The listing builds one solid part. Answer for the finished solid, in the listing's coordinates (mm). Face numbers are marked on the shaded views. A direction names the side the tool comes from. Coordinates: 2 decimals unless noted, no trailing zeros. Write each loop counter-clockwise with the first axis right and the second up, starting at its lowest first coordinate (ties: lowest second). Pieces come first, ordered by that corner, then holes.
(1) Given P1, Ø1, axis at y = -0.5, z = 6.5, coming from the +X side; P2, Ø6, axis at y = -5.5, z = 15, coming from the -X side; P3, Ø4, axis at x = 13, z = 8.5, coming from the +Y side, each flat-ended and moving along its own axis, determine where each tip first touches the part or whether it passes through.
(2) Which of the six approach directions +Z, -Z, +X, -X, +Y, -Y give full straight-line access (tool end or side, diameter ignored) to the marked faces 1 and 2?
(3) Straight lines are drawn through the part: line 1 (Y direction, x = 23.25, z = 12.5); line 2 (Y direction, x = 13, z = 4.75); line 3 (X direction, y = 11.5, z = 13.75). For each, find the intervals that lie inside material, in ascending order.
(4) The part is cut by section B-B on x = 23.75. Determine the outline of the cut face in (y, z).
(5) The part is cut by section A-A on z = 2.75. Determine the outline of the cut face in (x, y).
(6) The part is cut by section C-C on y = 12.5. Determine the outline of the cut face in (x, z), plus the area to 3 significant figures.
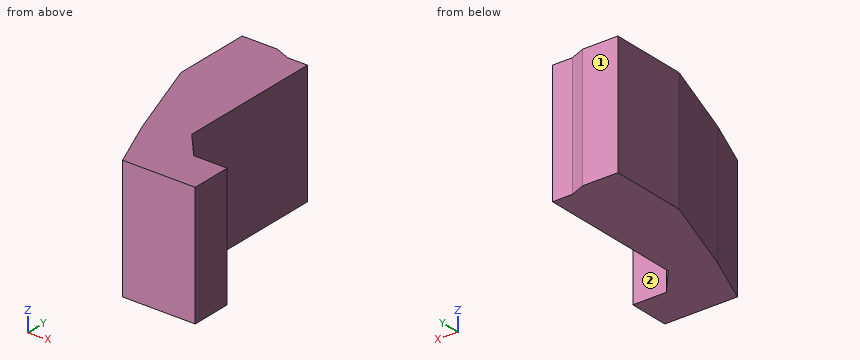
from build123d import *

# Parameters (mm, degrees)
PAD_DEPTH = 21


with BuildPart() as part:
    # Sketch → Pad (new body)
    with BuildSketch(Plane.XY):
        Polygon((15.064161, 13.763299), (15.064161, -11.529544), (19.077391, -16.168041), (24.861727, -16.168041), (24.861727, -23.168041), (12.321744, -23.168041), (8.41961, -13.925244), (2.937834, 1.476605), (2.937834, 14.82831), (9.042294, 14.82831), (11.646651, 13.763299), align=None)
    extrude(amount=PAD_DEPTH)


solid = part.part
Model answer:
1. P1: stops at x = 15.06
1. P2: stops at x = 4.35
1. P3: stops at y = 14.03
2. face 1: +Z, -Z, +X, -X, +Y
2. face 2: +Z, -Z, +X, +Y
3. line 1: y = -23.17 to -16.17
3. line 2: y = -23.17 to 13.76
3. line 3: x = 2.94 to 15.06
4. outline: (-23.17, 0) - (-16.17, 0) - (-16.17, 21) - (-23.17, 21) - close
5. outline: (2.94, 1.48) - (8.42, -13.93) - (12.32, -23.17) - (24.86, -23.17) - (24.86, -16.17) - (19.08, -16.17) - (15.06, -11.53) - (15.06, 13.76) - (11.65, 13.76) - (9.04, 14.83) - (2.94, 14.83) - close
6. outline: (2.94, 0) - (15.06, 0) - (15.06, 21) - (2.94, 21) - close
6. area: 255 mm2
